from build123d import *

# Parameters (mm, degrees)
SKETCH1_R           = 50.3
BOSS_EXTRUDE1_DEPTH = 6.35
CUT_EXTRUDE1_REACH  = 85.65
SKETCH2_R           = 1.15
CIRPATTERN1_COUNT   = 3
CUT_EXTRUDE2_REACH  = 85.65
SKETCH3_R           = 1.15


with BuildPart() as part:
    # Sketch1 → Boss-Extrude1 (new body)
    with BuildSketch(Plane(origin=(0, 0, 0), x_dir=(1, 0, 0), z_dir=(0, 1, 0))):
        with BuildLine():
            Line((-10, -53.87986637), (-10, -62.87986637))
            Line((-10, -62.87986637), (10, -62.87986637))
            Line((10, -62.87986637), (10, -53.87986637))
            ThreePointArc((10, -53.87986637), (0, 54.8), (-10, -53.87986637))
        make_face()
        with Locations(Location((0, 0, 0), (0, 0, 270))):
            Circle(SKETCH1_R, mode=Mode.SUBTRACT)
    extrude(amount=BOSS_EXTRUDE1_DEPTH)

    # Sketch2 → Cut-Extrude1 (cut, up to next)
    with BuildSketch(Plane(origin=(0, 6.35, 0), x_dir=(1, 0, 0), z_dir=(0, 1, 0)), mode=Mode.PRIVATE) as cut_extrude1_sk1:
        with Locations(Location((0, -52.55, 0), (0, 0, 270))):
            Circle(SKETCH2_R)
    cut_extrude1_tool1 = extrude(cut_extrude1_sk1.sketch, amount=-CUT_EXTRUDE1_REACH, mode=Mode.PRIVATE) & part.part
    cut_extrude1 = cut_extrude1_tool1.solids().sort_by_distance((0, 6.35, 52.55))[0]
    add(cut_extrude1, mode=Mode.SUBTRACT)

    # CirPattern1: Cut-Extrude1 ×3 about axis
    cirpattern1_axis = Axis((0, 0, 0), (0, 1, 0))
    for i in range(1, CIRPATTERN1_COUNT):
        add(cut_extrude1.rotate(cirpattern1_axis, i * 360 / CIRPATTERN1_COUNT), mode=Mode.SUBTRACT)

    # Sketch3 → Cut-Extrude2 (cut, up to next)
    with BuildSketch(Plane(origin=(0, 6.35, 0), x_dir=(1, 0, 0), z_dir=(0, 1, 0)), mode=Mode.PRIVATE) as cut_extrude2_sk1:
        with BuildLine():
            ThreePointArc((41.376904985, 35.930373417), (-47.56676712, 27.21107616), (-10, -53.87986637))
            Line((-10, -53.87986637), (-10, -49.295943038))
            ThreePointArc((-10, -49.295943038), (-43.451541655, 25.338775184), (37.979166437, 32.979886548))
            Line((37.979166437, 32.979886548), (41.376904985, 35.930373417))
        make_face()
        with Locations((-45.509634969, 26.275)):
            Circle(SKETCH3_R, mode=Mode.SUBTRACT)
    cut_extrude2_tool1 = extrude(cut_extrude2_sk1.sketch, amount=-CUT_EXTRUDE2_REACH, mode=Mode.PRIVATE) & part.part
    add(cut_extrude2_tool1.solids().sort_by_distance((-43.576908, 6.35, -25.411882))[0], mode=Mode.SUBTRACT)


solid = part.part
Can you work these out from the model? Positions are in its coordinate system, mm. A direction names the side the tool comes from. Give positions to 0.01 mm unless a question says otherwise; leave off trailing zeros. Order: outer loops, then holes, each group sorted by start corner. A loop starts at its lowest first (then second) coordinate and runs counter-clockwise, first axis right, second up. Notation, with made-up numbers: M 40,-25.75 L 45,-25.75 A32 cw 45,3.25 Z; hole C 78.25,-24 d2. An arc over 180 degrees is marked long. Use one line per item in the form item = value. Start each with the question number.
Item 1: We'd pull the mould along Z, two halves only. Please class faces 1 (the cylindrical face through (43, 3.1, 26.1)), 2 (the flat face through (-10, 3, 56)), 3 (the cylindrical face through (51.462, 3.131, 18.833)): +Z half, -Z half, draft (parallel to the pull), parting line (faces both ways), or undercut.
Item 2: Will these pins go through, and if not, where does the flat tip stop? pin 1 Ø2 at (y, z) = (4, 10.5) entering from +X; pin 2 Ø1.4 at (x, z) = (0, 52.55) entering from -Y.
Item 3: If we section it at C-C (y = 5): Write out the boundary of the cut face in (x, z) (3 decimals), then the cut area to 3 significant figures.
Item 4: If we section it at B-B (z = 52.55): Write out the boundary of the cut face in (x, y).
Item 5: If I drill on line 1 along Z through (x, y) = (45, 1); line 2 along X through (y, z) = (2, 0.5); line 3 along X through (y, z) = (2, -8), over which ranges is the centre line in solid material (lowest first)?
Item 6: If we section it at A-A (x = 0): Write out the boundary of the cut face in (y, z), then the cut area to 3 significant figures.
Item 7: If we section it at D-D (x = 7): Write out the boundary of the cut face in (y, z), then the cut area to 3 significant figures.
Item 8: For faces 4 (the cylindrical face through (44.387, 3.219, -26.524)), 5 (the flat face through (10, 3, 58)), which set-ups out of +Z, -Z, +X, -X, +Y, -Y let a thin tool reach every point of the face, with its end or its side?
Outcome:
q1.face_1 = undercut
q1.face_2 = draft
q1.face_3 = parting line
q2.pin_1 = 53.97
q2.pin_2 = through
q3.outline = M -10,49.296 A50.3 cw 37.979,-32.98 L 41.377,-35.93 A54.8 ccw 10,53.88 L 10,62.88 L -10,62.88 Z; hole C 0,52.55 d2.3; hole C 45.51,-26.275 d2.3
q3.area = 745 mm2
q4.outline = M -10,0 L -1.15,0 L -1.15,6.35 L -10,6.35 Z; M 1.15,0 L 15.54,0 L 15.54,6.35 L 1.15,6.35 Z
q5.line_1 = -31.27 to -27.31, -25.24 to -22.47, 22.47 to 31.27
q5.line_2 = 50.3 to 54.8
q5.line_3 = 49.66 to 54.21
q6.outline = M 0,50.3 L 6.35,50.3 L 6.35,51.4 L 0,51.4 Z; M 0,53.7 L 6.35,53.7 L 6.35,62.88 L 0,62.88 Z
q6.area = 65.3 mm2
q7.outline = M 0,49.81 L 6.35,49.81 L 6.35,62.88 L 0,62.88 Z
q7.area = 83.0 mm2
q8.face_4 = +Y, -Y
q8.face_5 = +Z, +X, +Y, -Y
